Build history of the part. All positions in model axes, mm. A direction names the side the tool comes from. Round coordinates to 2 decimals unless told otherwise and drop trailing zeros. Write each loop counter-clockwise with the first axis right and the second up, starting at its lowest first coordinate (ties: lowest second). Pieces come first, ordered by that corner, then holes.
from build123d import *

# Parameters (mm, degrees)
SKETCH1_W           = 57.3
SKETCH1_H           = 57.3
SKETCH1_R           = 3.175
SKETCH1_R_2         = 2.6
BOSS_EXTRUDE1_DEPTH = 76.5
SKETCH1_4_R         = 3.175
SKETCH1_4_R_2       = 2.925
BOSS_EXTRUDE2_DEPTH = 82.5
SKETCH1_5_R         = 2.925
BOSS_EXTRUDE3_DEPTH = 97.5


with BuildPart() as part:
    # Sketch1 → Boss-Extrude1 (new body)
    with BuildSketch(Plane(origin=(0, 0, 0), x_dir=(1, 0, 0), z_dir=(0, 1, 0))):
        with Locations((28.65, -28.65)):
            Rectangle(SKETCH1_W, SKETCH1_H)
        with Locations(Location((28.65, -28.65, 0), (0, 0, 270))):
            Circle(SKETCH1_R, mode=Mode.SUBTRACT)
        with Locations(Location((52.15, -52.15, 0), (0, 0, 270))):
            Circle(SKETCH1_R_2, mode=Mode.SUBTRACT)
        with Locations(Location((5.15, -52.15, 0), (0, 0, 270))):
            Circle(SKETCH1_R_2, mode=Mode.SUBTRACT)
        with Locations(Location((52.15, -5.15, 0), (0, 0, 270))):
            Circle(SKETCH1_R_2, mode=Mode.SUBTRACT)
        with Locations(Location((5.15, -5.15, 0), (0, 0, 270))):
            Circle(SKETCH1_R_2, mode=Mode.SUBTRACT)
    extrude(amount=BOSS_EXTRUDE1_DEPTH)

    # Sketch1_4 → Boss-Extrude2 (add)
    with BuildSketch(Plane(origin=(0, 0, 0), x_dir=(1, 0, 0), z_dir=(0, 1, 0))):
        with Locations(Location((28.65, -28.65, 0), (0, 0, 270))):
            Circle(SKETCH1_4_R)
        with Locations(Location((28.65, -28.65, 0), (0, 0, 270))):
            Circle(SKETCH1_4_R_2, mode=Mode.SUBTRACT)
    extrude(amount=BOSS_EXTRUDE2_DEPTH)

    # Sketch1_5 → Boss-Extrude3 (add)
    with BuildSketch(Plane(origin=(0, 0, 0), x_dir=(1, 0, 0), z_dir=(0, 1, 0))):
        with Locations(Location((28.65, -28.65, 0), (0, 0, 270))):
            Circle(SKETCH1_5_R)
    extrude(amount=BOSS_EXTRUDE3_DEPTH)


solid = part.part
1) Wall check: L1, parallel to Z at x = 5, y = 52.5; L2, parallel to X at y = 23, z = 50; L3, parallel to Y at x = 47.5, z = 22.5. Give the ranges that are in metal, low to high.
Results:
L1: z = 0 to 2.55, 7.75 to 49.55, 54.75 to 57.3
L2: x = 0 to 3.69, 6.61 to 50.69, 53.61 to 57.3
L3: y = 0 to 76.5
2) Slice it at A-A (y = 37.5). Write the cut outline in (x, z), plus the area to 3 significant figures.
Results:
outline: (0, 0) - (57.3, 0) - (57.3, 57.3) - (0, 57.3) - close; hole circle Ø5.2 at (5.15, 5.15); hole circle Ø5.2 at (5.15, 52.15); hole circle Ø5.2 at (52.15, 5.15); hole circle Ø5.2 at (52.15, 52.15)
area: 3,200 mm2
3) Which spindle directions (+Z, -Z, +X, -X, +Y, -Y) get a long thin tool onto all of the face, cutting with end or side? Do faces 5 (the cylindrical face through (54.728, 37.714, 51.812)), 6 (the cylindrical face through (31.8, 79.46, 28.24)). Say none if no direction does.
Results:
face 5: +Y, -Y
face 6: +Y
4) Mould opens along X. For faces 1 (the flat face through (57.3, 38, 29)), 2 (the flat face through (0, 38, 29)), 3 (the flat face through (28, 38, 0)), 4 (the cylindrical face through (54.728, 37.714, 4.812)) say: released by +X, released by -X, zero draft, split by the parting line, or undercut.
Results:
face 1: released by +X
face 2: released by -X
face 3: zero draft
face 4: undercut
5) Slice it at D-D (z = 28.65). Write the cut outline in (x, y) (3 decimals), plus the area to 3 significant figures.
Results:
outline: (0, 0) - (57.3, 0) - (57.3, 76.5) - (31.825, 76.5) - (31.825, 82.5) - (31.575, 82.5) - (31.575, 97.5) - (25.725, 97.5) - (25.725, 82.5) - (25.475, 82.5) - (25.475, 76.5) - (0, 76.5) - close
area: 4,510 mm2
6) Slice it at C-C (x = 52.15). Write the cut outline in (y, z), plus the area to 3 significant figures.
Results:
outline: (0, 0) - (76.5, 0) - (76.5, 2.55) - (0, 2.55) - close; (0, 7.75) - (76.5, 7.75) - (76.5, 49.55) - (0, 49.55) - close; (0, 54.75) - (76.5, 54.75) - (76.5, 57.3) - (0, 57.3) - close
area: 3,590 mm2
7) Pin check, flat tips, straight feed: pin 1 Ø4.5 at (x, z) = (5.15, 5.15) entering from -Y; pin 2 Ø3 at (y, z) = (44.5, 46) entering from -X; pin 3 Ø3 at (x, z) = (10.5, 40.5) entering from +Y. Stop position of each tip, or through.
Results:
pin 1: passes through
pin 2: stops at x = 0
pin 3: stops at y = 76.5
8) Slice it at B-B (z = 5.15). Write the cut outline in (x, y).
Results:
outline: (0, 0) - (2.55, 0) - (2.55, 76.5) - (0, 76.5) - close; (7.75, 0) - (49.55, 0) - (49.55, 76.5) - (7.75, 76.5) - close; (54.75, 0) - (57.3, 0) - (57.3, 76.5) - (54.75, 76.5) - close
